from build123d import *

# Parameters (mm, degrees)
F1_DEPTH  = 21.844
F5_R      = 9.3558336569
F6_DEPTH  = 58.42
F3_R      = 9.4583600755
F7_DEPTH  = 55.626
F4_R      = 9.3478497533
F8_DEPTH  = 52.832
F2_R      = 9.4635805484
F9_DEPTH  = 58.42
F12_R     = 31.3770390823
F10_R     = 31.5053231156
F11_R     = 31.5183409025
F13_R     = 31.5308798418
F14_DEPTH = 21.082
F21_D     = 6.35
F23_D     = 50.8
F25_D     = 50.8
F27_D     = 50.8
F29_D     = 50.8


# Not quite as in the source:
# - the program builds the solid bodies; features that only make, move or delete a surface that nothing else refers to are left out


with BuildPart() as f1:
    # F0 (on Front) → F1 (new body)
    with BuildSketch(Plane.XZ):
        Polygon((23.8739177585, 27.4659190327), (-27.4659190327, 23.8739177585), (-23.8739177585, -27.4659190327), (27.4659190327, -23.8739177585), align=None)
    extrude(amount=F1_DEPTH)

    # F5 (on face) → F6 (join)
    with BuildSketch(Plane(origin=(1.7960006371, 0, -25.6699183956), x_dir=(0.9975613857, 0, 0.0697945687), z_dir=(0.0697945687, 0, -0.9975613857))):
        with Locations((-3.9608110674, 10.7757570222)):
            Circle(F5_R)
    extrude(amount=F6_DEPTH)

    # F3 (on face) → F7 (join)
    with BuildSketch(Plane(origin=(25.6699183956, 0, 1.7960006371), x_dir=(0, 1, 0), z_dir=(0.9975613857, 0, 0.0697945687))):
        with Locations((-10.7757570222, 0)):
            Circle(F3_R)
    extrude(amount=F7_DEPTH)

    # F4 (on face) → F8 (join)
    with BuildSketch(Plane(origin=(-25.6699183956, 0, -1.7960006371), x_dir=(0, -1, 0), z_dir=(-0.9975613857, 0, -0.0697945687))):
        with Locations((10.5063626543, 3.6907584872)):
            Circle(F4_R)
    extrude(amount=F8_DEPTH)

    # F2 (on face) → F9 (join)
    with BuildSketch(Plane(origin=(-1.7960006371, 0, 25.6699183956), x_dir=(0.9975613857, 0, 0.0697945687), z_dir=(-0.0697945687, 0, 0.9975613857))):
        with Locations((0, -10.7757570222)):
            Circle(F2_R)
    extrude(amount=F9_DEPTH)

    # F12 (on Front) + F10 (on Front) + F11 (on Front) + F13 (on Front) → F14 (join)
    with BuildSketch(Plane.XZ):
        with Locations((81.530354917, 6.9857356139)):
            Circle(F12_R)
    with BuildSketch(Plane.XZ):
        with Locations((3.051524749, -84.1294080019)):
            Circle(F10_R)
    with BuildSketch(Plane.XZ):
        with Locations((-78.3801749349, 0)):
            Circle(F11_R)
    with BuildSketch(Plane.XZ):
        with Locations((-5.8717224747, 83.4135636687)):
            Circle(F13_R)
    extrude(amount=F14_DEPTH)

    # F21 (through all)
    with Locations(Plane(origin=(0, 0, 0), x_dir=(-1, 0, 0), z_dir=(0, 1, 0))):
        with Locations((23.8739177585, -27.4659190327), (-27.4659190327, -23.8739177585), (-23.8739177585, 27.4659190327), (27.4659190327, 23.8739177585)):
            Hole(F21_D / 2)

    # F23 (through all)
    with Locations(Plane(origin=(0, 0, 0), x_dir=(-1, 0, 0), z_dir=(0, 1, 0))):
        with Locations((5.8717224747, 83.4135636687)):
            Hole(F23_D / 2)

    # F25 (through all)
    with Locations(Plane(origin=(0, 0, 0), x_dir=(-1, 0, 0), z_dir=(0, 1, 0))):
        with Locations((-81.530354917, 6.9857356139)):
            Hole(F25_D / 2)

    # F27 (through all)
    with Locations(Plane(origin=(0, 0, 0), x_dir=(-1, 0, 0), z_dir=(0, 1, 0))):
        with Locations((78.3801749349, 0)):
            Hole(F27_D / 2)

    # F29 (through all)
    with Locations(Plane(origin=(0, 0, 0), x_dir=(-1, 0, 0), z_dir=(0, 1, 0))):
        with Locations((-3.051524749, -84.1294080019)):
            Hole(F29_D / 2)


solid = f1.part
Geometry: final body of the model. Coordinates: model frame, mm. A direction names the side the tool comes from. Give positions to 0.01 mm unless a question says otherwise; leave off trailing zeros. Write each loop counter-clockwise with the first axis right and the second up, starting at its lowest first coordinate (ties: lowest second). Pieces come first, ordered by that corner, then holes.
(1) Cut plane B-B, the plane x = 67. Return loops of the section in (y, z), then the cut area to 3 significant figures.
(2) First-contact query: P1, Ø3, axis at x = -77.5, y = -19.5, coming from the +Z side; P2, Ø4, axis at x = 76, y = -14.5, coming from the +Z side; P3, Ø10, axis at x = -36, y = -7.5, coming from the -Z side. Flat tips, straight axial feed; report the tip coordinate or a pass-through.
(3) Ray query, line 1 (Z direction, x = 0, y = -19.25); line 2 (Z direction, x = -23, y = -1.5); line 3 (Z direction, x = -15, y = -10.5). Return the intervals inside material, ascending.
(4) Cut plane D-D, the plane x = 16.5. Return loops of the section in (y, z), then the cut area to 3 significant figures.
(5) Cut plane A-A, the plane z = -75.5. Return loops of the section in (x, y).
(6) Mould query, pull axis X, two halves, no side actions, for faces 1 (the flat face through (-27, -21.082, 98)), 2 (the cylindrical face through (105.757, -10.689, 14.615)), 3 (the cylindrical face through (-3.778, -10.393, -114.886)). Classes: released by +X, released by -X, zero draft, split by the parting line, or undercut.
(7) Cut plane C-C, the plane y = -13.5. Return loops of the section in (x, z) (3 decimals).
(8) Access query for faces 4 (the cylindrical face through (39.34, -6.41, -5.66)), 5 (the flat face through (5, -21.082, -58)). Directions: +Z, -Z, +X, -X, +Y, -Y. A direction counts if a zero-diameter tool reaches every point of the face in a straight line with its end or side. Return the directions, or none.
Values follow:
1. outline: (-21.08, -20.82) - (0, -20.82) - (0, -13.85) - (-21.08, -13.85) - close; (-21.08, 27.82) - (0, 27.82) - (0, 34.8) - (-21.08, 34.8) - close
1. area: 294 mm2
2. P1: stops at z = 31.52
2. P2: stops at z = 38.16
2. P3: stops at z = -8.48
3. line 1: z = -115.49 to -109.35, -58.91 to 58.7, 108.13 to 114.39
3. line 2: z = -101.85 to -66.41, -24.41 to 24.19, 56.94 to 64.66, 102.17 to 109.89
3. line 3: z = -109.95 to -102, -66.26 to -58.31, -26.85 to 24.75, 53.23 to 59.71, 107.12 to 113.59
4. outline: (-21.84, -24.64) - (0, -24.64) - (0, 26.95) - (-21.84, 26.95) - close; (-21.08, -112.62) - (0, -112.62) - (0, -105.68) - (-21.08, -105.68) - close; (-21.08, -62.58) - (0, -62.58) - (0, -55.64) - (-21.08, -55.64) - close; (-21.08, 61.19) - (0, 61.19) - (0, 71.39) - (-21.08, 71.39) - close; (-21.08, 95.44) - (0, 95.44) - (0, 105.63) - (-21.08, 105.63) - close
4. area: 1,850 mm2
5. outline: (-27.25, -21.08) - (-20.84, -21.08) - (-20.84, 0) - (-27.25, 0) - close; (26.94, -21.08) - (33.35, -21.08) - (33.35, 0) - (26.94, 0) - close
6. face 1: zero draft
6. face 2: undercut
6. face 3: split by the parting line
7. outline: (-48.235, 9.202) arc R31.518 ccw (long way) to (-48.04, -8.539) - (-25.309, -6.948) - (-24.096, -24.299) arc R3.175 cw to (-20.707, -27.244) - (-11.084, -26.571) - (-9.091, -55.058) arc R31.505 ccw (long way) to (8.72, -53.138) - (6.773, -25.322) - (24.299, -24.096) arc R3.175 cw to (27.244, -20.707) - (26.302, -7.239) - (52.698, -5.393) arc R31.377 ccw (long way) to (50.664, 12.624) - (25.038, 10.831) - (24.096, 24.299) arc R3.175 cw to (20.707, 27.244) - (7.245, 26.302) - (5.312, 53.933) arc R31.531 ccw (long way) to (-12.769, 52.646) - (-10.837, 25.037) - (-24.299, 24.096) arc R3.175 cw to (-27.244, 20.707) - (-26.546, 10.72) - close; hole circle Ø50.8 at (-78.38, 0); hole circle Ø50.8 at (-5.872, 83.414); hole circle Ø50.8 at (3.052, -84.129); hole circle Ø50.8 at (81.53, 6.986)
8. face 4: none
8. face 5: -Z, +X, -X, -Y
